Could you check a few things on this model? Use its own coordinates, in mm. Face numbers are marked on the shaded views. A direction names the side the tool comes from. Round coordinates to 2 decimals unless told otherwise and drop trailing zeros. Order: outer loops, then holes, each group sorted by start corner. A loop starts at its lowest first (then second) coordinate and runs counter-clockwise, first axis right, second up. Notation, with made-up numbers: (-4.75, -2) -> (3.25, -2) arc R15 cw to (3.25, 2) -> close; hole circle Ø2 at (19, -27.75). An arc over 180 degrees is marked (long way). Put each result on its own line as item: value. Start each with the question number.
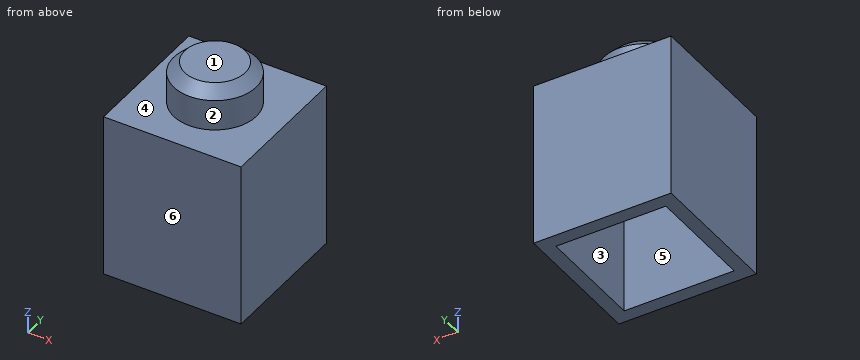
from build123d import *

# Parameters (mm, degrees)
F0_W     = 15.875
F0_H     = 15.875
F1_DEPTH = 9.525
F2_R     = 4.7625
F3_DEPTH = 4.826
F4_SIZE  = 1.27
F5_T     = -1.5875


with BuildPart() as f1:
    # F0 (on Top) → F1 (new body, symmetric)
    with BuildSketch(Plane.XY):
        Rectangle(F0_W, F0_H)
    extrude(amount=F1_DEPTH, both=True)

    # F2 (on face) → F3 (join)
    with BuildSketch(Plane.XY.offset(9.525)):
        Circle(F2_R)
    extrude(amount=F3_DEPTH)

    # F4
    f4_edges = [f1.edges().sort_by_distance(p)[0] for p in [
        (-4.7625, 0, 14.351),
    ]]
    chamfer(f4_edges, length=F4_SIZE)

    # F5
    f5_openings = [f1.faces().sort_by_distance(p)[0] for p in [
        (0, 0, -9.525),
    ]]
    offset(amount=F5_T, openings=f5_openings, kind=Kind.INTERSECTION)


solid = f1.part
1. Thinking about a two-plate mould opening in Y: for the marked faces 4, 5 and 6, which applies, +Y half, -Y half, draft (parallel to the pull), parting line (faces both ways), or undercut?
2. If we section it at A-A, the plane z = -2.5: Please give me the cut outline in (x, y), then the cut area to 3 significant figures.
3. I need wall thicknesses on L1, parallel to Y at x = 1, z = 5. Which ranges of the line are inside material? Lowest first, please.
4. Which directions (+Z, -Z, +X, -X, +Y, -Y) give clear straight access to the entire face, cutting with the end or side of a thin tool? Please do the marked faces 1, 2 and 3.
5. For pin 1 Ø4 at (x, y) = (0, 0) entering from -Z; pin 2 Ø6.5 at (x, y) = (-1, 0) entering from -Z, each with a flat end and sliding along its axis, tell me the tip position at first contact or that it passes through.
Results below:
1. face 4: draft
1. face 5: undercut
1. face 6: -Y half
2. outline: (-7.94, -7.94) -> (7.94, -7.94) -> (7.94, 7.94) -> (-7.94, 7.94) -> close; hole (-6.35, -6.35) -> (6.35, -6.35) -> (6.35, 6.35) -> (-6.35, 6.35) -> close
2. area: 90.7 mm2
3. L1: -7.94 to -6.35, 6.35 to 7.94
4. face 1: +Z, +X, -X, +Y, -Y
4. face 2: +Z
4. face 3: -Z
5. pin 1: z = 12.76
5. pin 2: z = 7.94
